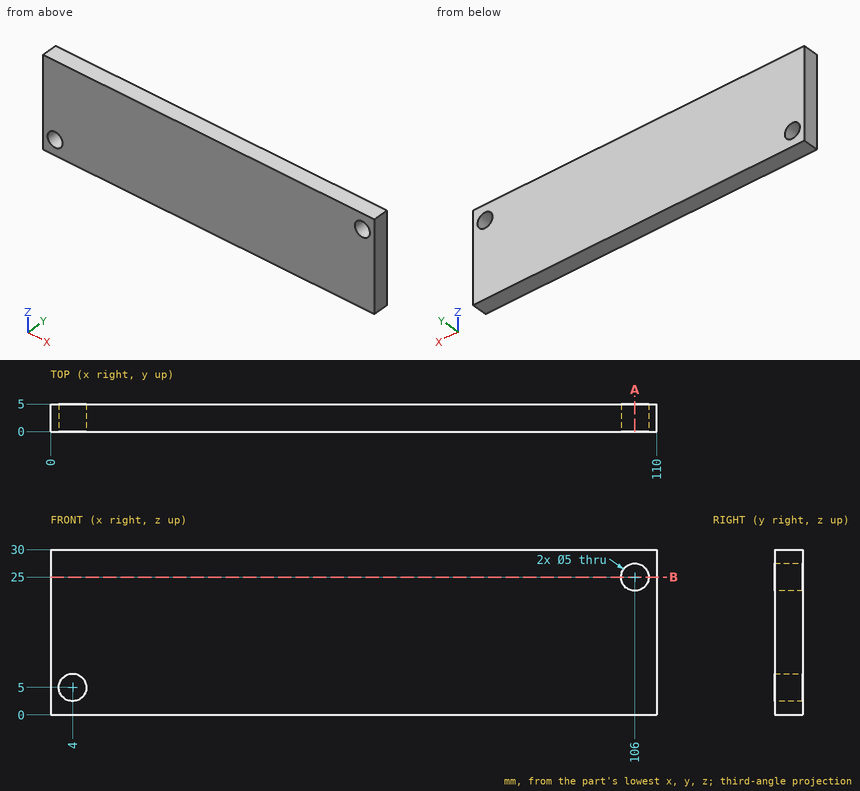
Answer from the drawing. Dimensions are ordinates in mm from the lowest x, y and z of the part. Coordinates: 2 decimals unless noted, no trailing zeros. Order: outer loops, then holes, each group sorted by start corner. A loop starts at its lowest first (then second) coordinate and runs counter-clockwise, first axis right, second up. Notation, with made-up numbers: (46, 47) - (65, 47) arc R21 cw to (65, 81) - close; hole circle Ø11 at (-21.75, 72.25). An arc over 180 degrees is marked (long way). Put each result on its own line as item: value. Start each with the question number.
1) A flat-ended cylindrical pin translates along its axis: pin 1 (4.5 mm diameter, centred on x = 106, z = 25, fed in from +Y). Find the tip coordinate at first contact, or state that the pin passes through.
2) Find the intervals of material crossed by line 1 (Z direction, x = 106, y = 2.25); line 2 (X direction, y = 3.45, z = 5); line 3 (X direction, y = 3.5, z = 25), in increasing order. Write a range as from..to.
3) Find section A-A (x = 106). Give the vertices of the cut face in (y, z), plus the area to 3 significant figures.
4) Find section B-B (z = 25). Give the vertices of the cut face in (x, y), plus the area to 3 significant figures.
Results list:
1. pin 1: passes through
2. line 1: z = 0..22.5, 27.5..30
2. line 2: x = 0..1.5, 6.5..110
2. line 3: x = 0..103.5, 108.5..110
3. outline: (0, 0) - (5, 0) - (5, 22.5) - (0, 22.5) - close; (0, 27.5) - (5, 27.5) - (5, 30) - (0, 30) - close
3. area: 125 mm^2
4. outline: (0, 0) - (103.5, 0) - (103.5, 5) - (0, 5) - close; (108.5, 0) - (110, 0) - (110, 5) - (108.5, 5) - close
4. area: 525 mm^2
